```python
from build123d import *

# Parameters (mm, degrees)
SKETCH_1_R          = 1.5
SKETCH_1_R_2        = 30
SKETCH_1_W          = 4.4
SKETCH_1_H          = 8.4
EXTRUDE_1_DEPTH     = 4
SKETCH_4_R          = 1.5
CUT_EXTRUDE_1_DEPTH = 10


with BuildPart() as part:
    # 草图1 → 凸台-拉伸1 (new body)
    with BuildSketch(Plane.XY):
        Polygon((0, 0), (0, -4), (-1.35, -4), (-1.35, -6.6), (0, -6.6), (0, -8.6), (3, -8.6), (3, -6.6), (4.35, -6.6), (4.35, -4), (3, -4), (3, 0), (30.5, 0), (30.5, 4), (38.5, 4), (38.5, 0), (66, 0), (66, -4), (64.65, -4), (64.65, -6.6), (66, -6.6), (66, -8.6), (69, -8.6), (69, -6.6), (70.35, -6.6), (70.35, -4), (69, -4), (69, 0), (96.5, 0), (96.5, 4), (104.5, 4), (104.5, 0), (132, 0), (143.5, 0), (145.5, 0), (150.5, 0), (150.5, -200), (145.5, -200), (143.5, -200), (132, -200), (104.5, -200), (104.5, -204), (96.5, -204), (96.5, -200), (69, -200), (69, -196), (70.35, -196), (70.35, -193.4), (69, -193.4), (69, -191.4), (66, -191.4), (66, -193.4), (64.65, -193.4), (64.65, -196), (66, -196), (66, -200), (38.5, -200), (38.5, -204), (30.5, -204), (30.5, -200), (3, -200), (3, -196), (4.35, -196), (4.35, -193.4), (3, -193.4), (3, -191.4), (0, -191.4), (0, -193.4), (-1.35, -193.4), (-1.35, -196), (0, -196), (0, -200), (-27.5, -200), (-27.5, -204), (-35.5, -204), (-35.5, -200), (-63, -200), (-63, -196), (-61.65, -196), (-61.65, -193.4), (-63, -193.4), (-63, -191.4), (-66, -191.4), (-66, -193.4), (-67.35, -193.4), (-67.35, -196), (-66, -196), (-66, -200), (-93.5, -200), (-93.5, -204), (-101.5, -204), (-101.5, -200), (-129, -200), (-140.5, -200), (-142.5, -200), (-147.5, -200), (-147.5, 0), (-142.5, 0), (-140.5, 0), (-129, 0), (-101.5, 0), (-101.5, 4), (-93.5, 4), (-93.5, 0), (-66, 0), (-66, -4), (-67.35, -4), (-67.35, -6.6), (-66, -6.6), (-66, -8.6), (-63, -8.6), (-63, -6.6), (-61.65, -6.6), (-61.65, -4), (-63, -4), (-63, 0), (-35.5, 0), (-35.5, 4), (-27.5, 4), (-27.5, 0), align=None)
        with Locations((-142.5, -100)):
            Circle(SKETCH_1_R, mode=Mode.SUBTRACT)
        with Locations(Location((145.5, -100, 0), (0, 0, 180))):
            Circle(SKETCH_1_R, mode=Mode.SUBTRACT)
        with Locations((1.5, -100)):
            Circle(SKETCH_1_R_2, mode=Mode.SUBTRACT)
        with Locations((-142.5, -67)):
            Rectangle(SKETCH_1_W, SKETCH_1_H, mode=Mode.SUBTRACT)
        with Locations((-142.5, -133)):
            Rectangle(SKETCH_1_W, SKETCH_1_H, mode=Mode.SUBTRACT)
        with Locations((145.5, -133)):
            Rectangle(SKETCH_1_W, SKETCH_1_H, mode=Mode.SUBTRACT)
        with Locations((145.5, -67)):
            Rectangle(SKETCH_1_W, SKETCH_1_H, mode=Mode.SUBTRACT)
    extrude(amount=EXTRUDE_1_DEPTH)

    # 草图4 → 切除-拉伸1 (cut)
    with BuildSketch(Plane.XY.offset(4)):
        with Locations((-100.464854909, -102.524202067)):
            Circle(SKETCH_4_R)
        with Locations((-72.564854909, -102.524202067)):
            Circle(SKETCH_4_R)
        with Locations((-112.964854909, -153.324202067)):
            Circle(SKETCH_4_R)
        with Locations((-67.464854909, -154.624202067)):
            Circle(SKETCH_4_R)
        with Locations((-117.464854909, -35.441983185)):
            Circle(SKETCH_4_R)
        with Locations((-68.464854909, -35.441983185)):
            Circle(SKETCH_4_R)
        with Locations((-117.464854909, -93.441983185)):
            Circle(SKETCH_4_R)
        with Locations((-68.464854909, -93.441983185)):
            Circle(SKETCH_4_R)
    extrude(amount=-CUT_EXTRUDE_1_DEPTH, mode=Mode.SUBTRACT)


solid = part.part
```
Could you check a few things on this model? Use its own coordinates, in mm. Round coordinates to 2 decimals unless told otherwise and drop trailing zeros. Write each loop counter-clockwise with the first axis right and the second up, starting at its lowest first coordinate (ties: lowest second). Pieces come first, ordered by that corner, then holes. Notation, with made-up numbers: M 53.25,-10.5 L 60.25,-10.5 A38 cw 60.25,28.5 Z; hole C 26,32 d2. An arc over 180 degrees is marked long. Answer in a Markdown table with one row per item. Add a question column.
Q1. If we mould it in two halves opening along Y, with no side actions, what happens to faces 1 (the flat face through (-30, -99, 0)), 2 (the cylindrical face through (-2.405, -70.255, 1.972))? For each: +Y half, -Y half, draft (parallel to the pull), parting line (faces both ways), or undercut.
Q2. Will these pins go through, and if not, where does the flat tip stop? pin 1 Ø0.7 at (x, z) = (-1, 1.5) entering from +Y; pin 2 Ø2 at (x, z) = (-124, 1.5) entering from -Y; pin 3 Ø3.5 at (x, y) = (-100.46, -102.52) entering from +Z; pin 4 Ø1.2 at (y, z) = (3, 3) entering from +X.
Q3. Imagine slicing it at A-A (y = -84). Please give me the cut outline in (x, z), then the cut area to 3 significant figures.
Q4. If I drill on line 1 (X direction, y = -65.5, z = 3.2); line 2 (X direction, y = -195, z = 0.25); line 3 (X direction, y = -7.5, z = 3.7), over which ranges is the centre line in solid material (lowest first)? Write a range as from..to.
Q5. Imagine slicing it at B-B (x = 122). Please give me the cut outline in (y, z).
Q6. Imagine slicing it at C-C (z = 3.3). Give the number of separate pieces and of enclosed holes in the cut face, then the cut area to 3 significant figures.
Values:
| question | item | result |
|---|---|---|
| 1 | face 1 | draft |
| 1 | face 2 | undercut |
| 2 | pin 1 | y = 0 |
| 2 | pin 2 | y = -200 |
| 2 | pin 3 | z = 4 |
| 2 | pin 4 | x = 104.5 |
| 3 | outline | M -147.5,0 L -23.88,0 L -23.88,4 L -147.5,4 Z; M 26.88,0 L 150.5,0 L 150.5,4 L 26.88,4 Z |
| 3 | area | 989 mm^2 |
| 4 | line 1 | -147.5..-144.7, -140.3..143.3, 147.7..150.5 |
| 4 | line 2 | -147.5..-67.35, -61.65..-1.35, 4.35..64.65, 70.35..150.5 |
| 4 | line 3 | -147.5..-66, -63..0, 3..66, 69..150.5 |
| 5 | outline | M -200,0 L 0,0 L 0,4 L -200,4 Z |
| 6 | separate pieces | 1 |
| 6 | enclosed holes | 15 |
| 6 | area | 56,600 mm^2 |
